Design review of the part built by this model. Coordinates are the model's own, in mm. Face numbers are marked on the shaded views. A direction names the side the tool comes from. Give positions to 0.01 mm unless a question says otherwise; leave off trailing zeros. Write each loop counter-clockwise with the first axis right and the second up, starting at its lowest first coordinate (ties: lowest second). Pieces come first, ordered by that corner, then holes. Notation, with made-up numbers: M 63,18.5 L 83,18.5 A18 ccw 83,30.5 Z; hole C 4.25,82 d2. An arc over 180 degrees is marked long. Use one line per item in the form item = value. Start each with the question number.
from build123d import *

# Parameters (mm, degrees)
SKETCH1_W           = 14
SKETCH1_H           = 13
BOSS_EXTRUDE1_DEPTH = 10.1
SKETCH2_W           = 3.5
SKETCH2_H           = 3
BOSS_EXTRUDE2_DEPTH = 1.3
CUT_EXTRUDE1_REACH  = 11.5
SKETCH4_W           = 6.77
SKETCH4_H           = 5
BOSS_EXTRUDE3_DEPTH = 4.6
SKETCH5_W           = 6.77
SKETCH5_H           = 5
BOSS_EXTRUDE4_DEPTH = 4.6
SKETCH6_W           = 3.8
SKETCH6_H           = 3.8
CUT_EXTRUDE2_DEPTH  = 9.2
SKETCH7_W           = 1.094306831
SKETCH7_H           = 1.09430683
SKETCH7_W_2         = 1.09430683
BOSS_EXTRUDE5_DEPTH = 10
SKETCH7_4_W         = 1.094306831
SKETCH7_4_H         = 1.09430683
SKETCH7_4_W_2       = 1.09430683
SKETCH10_W          = 1.09430683
SKETCH10_H          = 1.09
SKETCH10_W_2        = 1.077227458
SKETCH10_H_2        = 1.094306831
SKETCH10_W_3        = 1.09
SKETCH10_2_W        = 1.09430683
SKETCH10_2_H        = 1.09
SKETCH10_2_W_2      = 1.077227458
SKETCH10_2_H_2      = 1.094306831
SKETCH10_2_W_3      = 1.09
BOSS_EXTRUDE6_DEPTH = 10
SKETCH12_R          = 1.2
CUT_EXTRUDE3_DEPTH  = 12.4


with BuildPart() as part:
    # Sketch1 → Boss-Extrude1 (new body)
    with BuildSketch(Plane(origin=(0, 0, 0), x_dir=(1, 0, 0), z_dir=(0, 1, 0))):
        with Locations((7, 6.5)):
            Rectangle(SKETCH1_W, SKETCH1_H)
    extrude(amount=BOSS_EXTRUDE1_DEPTH)

    # Sketch2 → Boss-Extrude2 (add)
    with BuildSketch(Plane(origin=(0, 10.1, 0), x_dir=(1, 0, 0), z_dir=(0, 1, 0))):
        with Locations((7.75, 1.5)):
            Rectangle(SKETCH2_W, SKETCH2_H)
    extrude(amount=BOSS_EXTRUDE2_DEPTH)

    # Sketch3 → Cut-Extrude1 (cut, up to next)
    with BuildSketch(Plane(origin=(9.5, 0, 0), x_dir=(0, 0, -1), z_dir=(1, 0, 0)), mode=Mode.PRIVATE) as cut_extrude1_sk1:
        Polygon((0, 10.1), (3, 11.4), (0, 11.4), align=None)
    cut_extrude1_tool1 = extrude(cut_extrude1_sk1.sketch, amount=-CUT_EXTRUDE1_REACH, mode=Mode.PRIVATE) & part.part
    add(cut_extrude1_tool1.solids().sort_by_distance((9.5, 10.966667, -1))[0], mode=Mode.SUBTRACT)

    # Sketch4 → Boss-Extrude3 (add)
    with BuildSketch(Plane(origin=(14, 0, 0), x_dir=(0, 0, -1), z_dir=(1, 0, 0))):
        with Locations((9.615, 2.5)):
            Rectangle(SKETCH4_W, SKETCH4_H)
    extrude(amount=BOSS_EXTRUDE3_DEPTH)

    # Sketch5 → Boss-Extrude4 (add)
    with BuildSketch(Plane.ZY):
        with Locations((-9.615, 2.5)):
            Rectangle(SKETCH5_W, SKETCH5_H)
    extrude(amount=BOSS_EXTRUDE4_DEPTH)

    # Sketch6 → Cut-Extrude2 (cut)
    with BuildSketch(Plane.XY):
        with Locations((3.054030332, 7.029063078)):
            Rectangle(SKETCH6_W, SKETCH6_H)
        with Locations((11.054030332, 3.029063078)):
            Rectangle(SKETCH6_W, SKETCH6_H)
        with Locations((11.054030332, 7.029063078)):
            Rectangle(SKETCH6_W, SKETCH6_H)
        with Locations((3.054030332, 3.029063078)):
            Rectangle(SKETCH6_W, SKETCH6_H)
        with Locations((7.054030332, 7.029063078)):
            Rectangle(SKETCH6_W, SKETCH6_H)
        with Locations((7.054030332, 3.029063078)):
            Rectangle(SKETCH6_W, SKETCH6_H)
    extrude(amount=-CUT_EXTRUDE2_DEPTH, mode=Mode.SUBTRACT)

    # Sketch7 → Boss-Extrude5 (add)
    with BuildSketch(Plane(origin=(0, 0, -13), x_dir=(-1, 0, 0), z_dir=(0, 0, -1))):
        with Locations((-11.035767077, 7.313802256)):
            Rectangle(SKETCH7_W, SKETCH7_H)
        with Locations((-7.041460246, 7.313802256)):
            Rectangle(SKETCH7_W_2, SKETCH7_H)
        with Locations((-3.047153416, 7.313802256)):
            Rectangle(SKETCH7_W, SKETCH7_H)
    extrude(amount=-BOSS_EXTRUDE5_DEPTH)

    # Sweep2: sweep along a path in Sketch8
    with BuildLine(Plane(origin=(4, 0, 0), x_dir=(0, 0, -1), z_dir=(1, 0, 0))) as sweep2_path:
        Line((13, 7.313802256), (17.025339082, 7.313802256))
        ThreePointArc((17.025339082, 7.313802256), (18.775188598, 6.588990854), (19.5, 4.839141338))
        Line((19.5, 4.839141338), (19.5, 0))
        Line((19.5, 0), (19.5, -3.6))
    # Sketch7_4 → Sweep2 (sweep)
    with BuildSketch(Plane(origin=(0, 0, -13), x_dir=(-1, 0, 0), z_dir=(0, 0, -1))):
        with Locations((-11.035767077, 7.313802256)):
            Rectangle(SKETCH7_4_W, SKETCH7_4_H)
        with Locations((-7.041460246, 7.313802256)):
            Rectangle(SKETCH7_4_W_2, SKETCH7_4_H)
        with Locations((-3.047153416, 7.313802256)):
            Rectangle(SKETCH7_4_W, SKETCH7_4_H)
    sweep(path=sweep2_path.line)

    # Sweep3: sweep along a path in Sketch11
    with BuildLine(Plane(origin=(4, 0, 0), x_dir=(0, 0, -1), z_dir=(1, 0, 0))) as sweep3_path:
        Line((14, -3.6), (14, 0))
        Line((14, 0), (14, 1.79191881))
        ThreePointArc((14, 1.79191881), (13.707106781, 2.499025591), (13, 2.79191881))
    # Sketch10 → Sweep3 (sweep)
    with BuildSketch(Plane(origin=(0, 0, -13), x_dir=(-1, 0, 0), z_dir=(0, 0, -1))):
        with Locations((-3.0642338, 2.79191881)):
            Rectangle(SKETCH10_W, SKETCH10_H)
        with Locations((-7.049999932, 2.789495426)):
            Rectangle(SKETCH10_W_2, SKETCH10_H_2)
        with Locations((-11.033613661, 2.789495426)):
            Rectangle(SKETCH10_W_3, SKETCH10_H_2)
    sweep(path=sweep3_path.line)

    # Sketch10_2 → Boss-Extrude6 (add)
    with BuildSketch(Plane(origin=(0, 0, -13), x_dir=(-1, 0, 0), z_dir=(0, 0, -1))):
        with Locations((-3.0642338, 2.79191881)):
            Rectangle(SKETCH10_2_W, SKETCH10_2_H)
        with Locations((-7.049999932, 2.789495426)):
            Rectangle(SKETCH10_2_W_2, SKETCH10_2_H_2)
        with Locations((-11.033613661, 2.789495426)):
            Rectangle(SKETCH10_2_W_3, SKETCH10_2_H_2)
    extrude(amount=-BOSS_EXTRUDE6_DEPTH)

    # Sketch12 → Cut-Extrude3 (cut, through all)
    with BuildSketch(Plane.XZ):
        with Locations((-1.4, -10.4)):
            Circle(SKETCH12_R)
        with Locations((15.4, -10.4)):
            Circle(SKETCH12_R)
    extrude(amount=-CUT_EXTRUDE3_DEPTH, mode=Mode.SUBTRACT)


solid = part.part
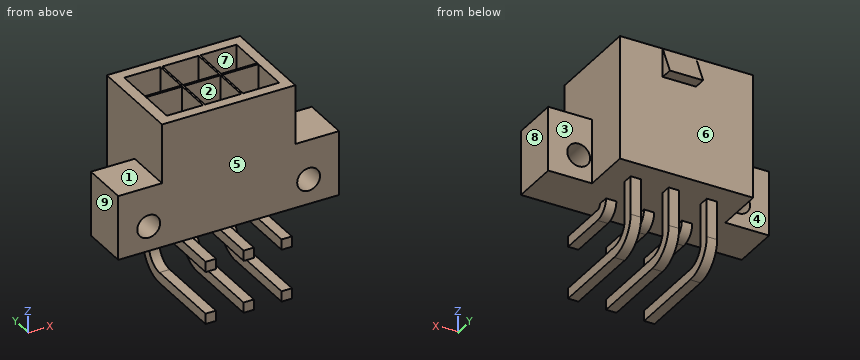
1. We need section B-B (x = 15.4). State the section outline as (y, z) points.
2. We need section C-C (y = -1.75). State the section outline as (x, z) points (3 decimals).
3. For the marked faces 1, 2, 3, 4 and 5, list the 3-axis set-ups (+Z, -Z, +X, -X, +Y, -Y) from which the entire face can be reached by the end or side of a thin tool; tool diameter is ignored.
4. Clearance check with flat-ended pins moving along their axes: pin 1 Ø5 at (x, z) = (-2, -9.5) entering from +Y; pin 2 Ø0.8 at (y, z) = (1.5, -13.5) entering from -X; pin 3 Ø0.9 at (x, z) = (11, -14.5) entering from +Y. State where each tip first meets the part, or that it passes through.
5. Draft analysis for pull direction X (two halves, no side actions). For the marked faces 6, 7, 8 and 9, state which applies: pulls with the +X half, pulls with the -X half, needs draft (parallel to the pull), parting line crosses it, or undercut.
6. We need section D-D (z = -5.5). Give the number of separate pieces and of enclosed holes in the cut face, and give its area (3 significant figures).
7. We need section A-A (z = -10.4). State the section outline as (x, y) points.
8. To check wall thickness, follow L1, parallel to Y at x = 12.25, z = -8.75; L2, parallel to X at y = 1.25, z = -5.5; L3, parallel to X at y = 2.75, z = -9.5. State the ranges of each line that lie inside material, in increasing order.
Answer block:
q1.outline = M 0,-13 L 5,-13 L 5,-11.6 L 0,-11.6 Z; M 0,-9.2 L 5,-9.2 L 5,-6.23 L 0,-6.23 Z
q2.outline = M 2.5,-20.047 L 3.594,-20.047 L 3.594,-18.953 L 2.5,-18.953 Z; M 2.517,-14.545 L 3.611,-14.545 L 3.611,-13.455 L 2.517,-13.455 Z; M 6.494,-20.047 L 7.589,-20.047 L 7.589,-18.953 L 6.494,-18.953 Z; M 6.511,-14.545 L 7.589,-14.545 L 7.589,-13.45 L 6.511,-13.45 Z; M 10.489,-20.047 L 11.583,-20.047 L 11.583,-18.953 L 10.489,-18.953 Z; M 10.489,-14.545 L 11.579,-14.545 L 11.579,-13.45 L 10.489,-13.45 Z
q3.face_1 = +Z, -X, +Y, -Y
q3.face_2 = +Z
q3.face_3 = +Z, -Z, +X, +Y
q3.face_4 = +Z, -Z, -X, +Y
q3.face_5 = +Z, +X, -X, -Y
q4.pin_1 = 10.1
q4.pin_2 = 2.52
q4.pin_3 = 7.86
q5.face_6 = needs draft
q5.face_7 = undercut
q5.face_8 = pulls with the +X half
q5.face_9 = pulls with the -X half
q6.separate_pieces = 7
q6.enclosed_holes = 6
q6.area = 61.9 mm^2
q7.outline = M -4.6,0 L -2.6,0 L -2.6,5 L -4.6,5 Z; M -0.2,0 L 14.2,0 L 14.2,5 L 14,5 L 14,10.1 L 0,10.1 L 0,5 L -0.2,5 Z; M 16.6,0 L 18.6,0 L 18.6,5 L 16.6,5 Z
q8.L1 = 0 to 1.13, 4.93 to 5.13, 8.93 to 10.1
q8.L2 = 0 to 1.15, 4.95 to 5.15, 8.95 to 9.15, 12.95 to 14
q8.L3 = -4.6 to -2.19, -0.61 to 14.61, 16.19 to 18.6
